For this review, take the finished solid that the model builds, in its own axes (mm). Face numbers are marked on the shaded views. A direction names the side the tool comes from. Give positions to 0.01 mm unless a question says otherwise; leave off trailing zeros. Loops run counter-clockwise (first coordinate to the right, second up) from the corner with the lowest first, then second, coordinate; pieces in that order, holes last. Notation, with made-up numbers: M 74,80 L 121,80 A5 cw 121,85 Z; hole C -34,49 d1. An arc over 180 degrees is marked long. Use CSV: the item, a comma, the result in double quotes. Start each with the question number.
1. To check wall thickness, follow line 1 (Z direction, x = -52, y = 8); line 2 (X direction, y = 31, z = 1.75); line 3 (X direction, y = 29.5, z = -1). State the ranges of each line that lie inside material, in increasing order. Write a range as [from, to].
2. Insertion check: P1, Ø3, axis at x = 52, z = -2, coming from the +Y side; P2, Ø4, axis at y = 21, z = 0.5, coming from the +X side; P3, Ø4, axis at x = 3.5, z = 3, coming from the -Y side. Each pin has a flat end and moves straight along its axis. Give the tip position at first contact, or say it passes through.
3. Take a section at C-C, the plane y = 10.5. Write out the cut boundary in (x, z), and give its area (3 significant figures).
4. Take a section at B-B, the plane z = -1.25. Write out the cut boundary in (x, y), and give its area (3 significant figures).
5. Tool access review of the marked faces 4, 5 and 6: name each direction out of +Z, -Z, +X, -X, +Y, -Y from which nothing blocks a thin tool from reaching the whole face with its end or side.
6. The part is to be moulded in two halves that separate along Y. For the marked faces 1, 2 and 3, say which applies: pulls with the +Y half, pulls with the -Y half, needs draft (parallel to the pull), parting line crosses it, or undercut.
7. Take a section at A-A, the plane x = -52. Write out the cut boundary in (y, z), and give its area (3 significant figures).
8. Take a section at D-D, the plane y = 21.5. Write out the cut boundary in (x, z).
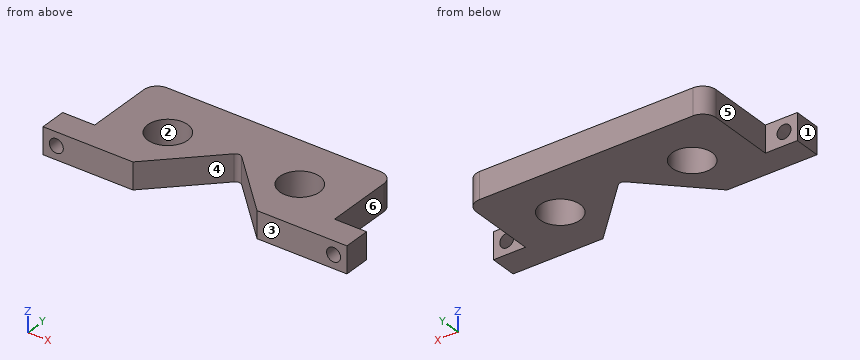
from build123d import *

# Parameters (mm, degrees)
SKETCH_1_R          = 7.5
EXTRUDE_1_DEPTH     = 5
SKETCH_2_R          = 2.612095194
CUT_EXTRUDE_1_DEPTH = 41


with BuildPart() as part:
    # 草圖1 → 填料-伸長1 (new body, symmetric)
    with BuildSketch(Plane.XY):
        with BuildLine():
            Line((-57, 15), (-57, 5))
            Line((-57, 5), (-23.284271247, 5))
            Line((-23.284271247, 5), (-1.414213562, 26.870057685))
            ThreePointArc((-1.414213562, 26.870057685), (0, 27.455844123), (1.414213562, 26.870057685))
            Line((1.414213562, 26.870057685), (23.284271247, 5))
            Line((23.284271247, 5), (57, 5))
            Line((57, 5), (57, 15))
            Line((57, 15), (45, 15))
            Line((45, 15), (45, 40))
            ThreePointArc((45, 40), (43.535533906, 43.535533906), (40, 45))
            Line((40, 45), (-40, 45))
            ThreePointArc((-40, 45), (-43.535533906, 43.535533906), (-45, 40))
            Line((-45, 40), (-45, 15))
            Line((-45, 15), (-57, 15))
        make_face()
        with Locations((-24.748737342, 24.748737342)):
            Circle(SKETCH_1_R, mode=Mode.SUBTRACT)
        with Locations((24.748737342, 24.748737342)):
            Circle(SKETCH_1_R, mode=Mode.SUBTRACT)
    extrude(amount=EXTRUDE_1_DEPTH, both=True)

    # 草圖2 → 除料-伸長1 (cut, through all)
    with BuildSketch(Plane.XZ.offset(-5)):
        with Locations((-52, 0)):
            Circle(SKETCH_2_R)
        with Locations((52, 0)):
            Circle(SKETCH_2_R)
    extrude(amount=-CUT_EXTRUDE_1_DEPTH, mode=Mode.SUBTRACT)


solid = part.part
Result set:
1,line 1,"[-5, -2.61], [2.61, 5]"
1,line 2,"[-45, -28.89], [-20.6, 20.6], [28.89, 45]"
1,line 3,"[-45, -30.55], [-18.95, 18.95], [30.55, 45]"
2,P1,"y = 15"
2,P2,"x = 45"
2,P3,"y = 22.78"
3,outline,"M -57,-5 L -17.78,-5 L -17.78,5 L -57,5 Z; M 17.78,-5 L 57,-5 L 57,5 L 17.78,5 Z; hole C -52,0 d5.22; hole C 52,0 d5.22"
3,area,"741 mm2"
4,outline,"M -57,5 L -54.29,5 L -54.29,15 L -57,15 Z; M -49.71,5 L -23.28,5 L -1.41,26.87 A2 cw 1.41,26.87 L 23.28,5 L 49.71,5 L 49.71,15 L 45,15 L 45,40 A5 ccw 40,45 L -40,45 A5 ccw -45,40 L -45,15 L -49.71,15 Z; M 54.29,5 L 57,5 L 57,15 L 54.29,15 Z; hole C -24.75,24.75 d15; hole C 24.75,24.75 d15"
4,area,"2,840 mm2"
5,face 4,"+Z, -Z, -Y"
5,face 5,"+Z, -Z, -X, +Y"
5,face 6,"+Z, -Z, +X, +Y"
6,face 1,"needs draft"
6,face 2,"undercut"
6,face 3,"pulls with the -Y half"
7,outline,"M 5,-5 L 15,-5 L 15,-2.61 L 5,-2.61 Z; M 5,2.61 L 15,2.61 L 15,5 L 5,5 Z"
7,area,"47.8 mm2"
8,outline,"M -45,-5 L -31.51,-5 L -31.51,5 L -45,5 Z; M -17.99,-5 L -6.78,-5 L -6.78,5 L -17.99,5 Z; M 6.78,-5 L 17.99,-5 L 17.99,5 L 6.78,5 Z; M 31.51,-5 L 45,-5 L 45,5 L 31.51,5 Z"
